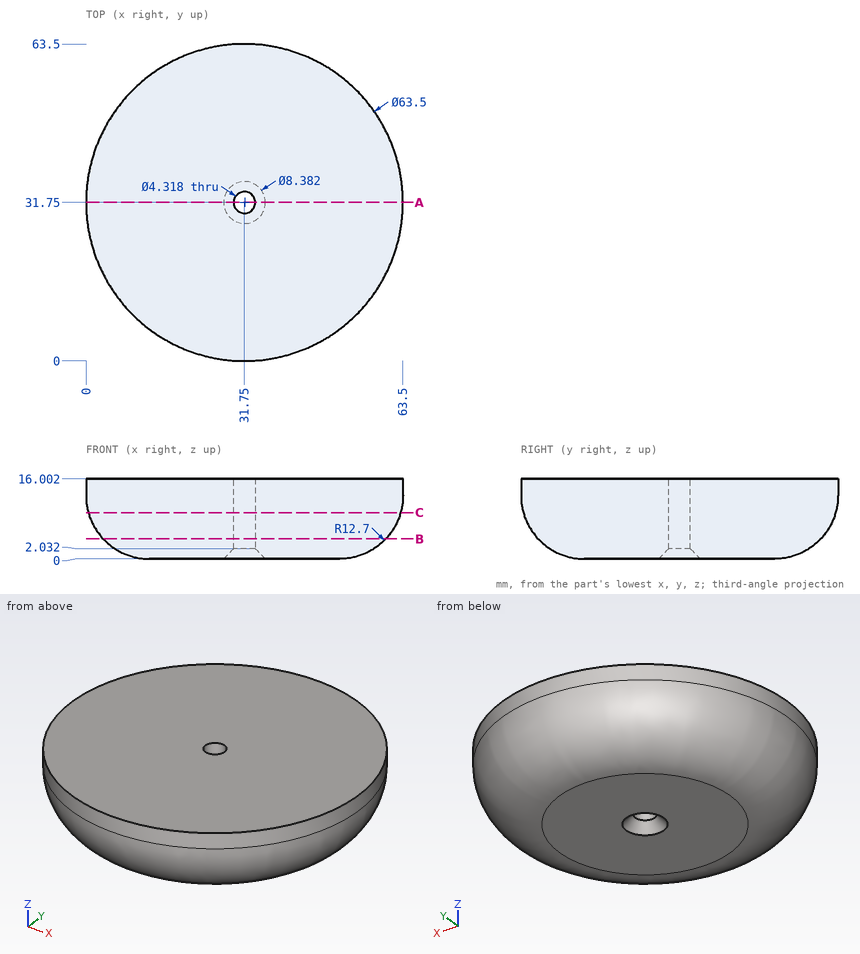
Answer from the drawing. Dimensions are ordinates in mm from the lowest x, y and z of the part. Give positions to 0.01 mm unless a question says otherwise; leave off trailing zeros. Loops run counter-clockwise (first coordinate to the right, second up) from the corner with the lowest first, then second, coordinate; pieces in that order, holes last. Notation, with made-up numbers: (-36.5, 44) -> (-4.5, 44) arc R15 cw to (-4.5, 62) -> close; hole circle Ø7 at (-35.75, 79). An arc over 180 degrees is marked (long way). Use a Markdown table: item, result.
Q1. Section B-B, the plane z = 4 is taken. Determine the outline of the cut face in (x, y), then the cut area to 3 significant figures.
Solved:
| item | result |
|---|---|
| outline | circle Ø56.6 at (31.75, 31.75); hole circle Ø4.32 at (31.75, 31.75) |
| area | 2,500 mm^2 |
Q2. Each of these flat-tipped pins is pushed along its axis until it touches: pin 1 (8 mm diameter, centred on x = 38.5, z = 2.5, fed in from +Y); pin 2 (8 mm diameter, centred on y = 21, z = 14, fed in from +X); pin 3 (3 mm diameter, centred on x = 9.5, y = 30, fed in from -Z). Where does it stop, or does it pass through?
Solved:
| item | result |
|---|---|
| pin 1 | stops at y = 61.26 |
| pin 2 | stops at x = 62.77 |
| pin 3 | stops at z = 0.12 |
Q3. Find the intervals of material crossed by line 1 along Y through (x, z) = (31.75, 12.5); line 2 along Y through (x, z) = (31.75, 6); line 3 along Z through (x, y) = (24, 5), in increasing order.
Solved:
| item | result |
|---|---|
| line 1 | y = 0 to 29.59, 33.91 to 63.5 |
| line 2 | y = 1.91 to 29.59, 33.91 to 61.59 |
| line 3 | z = 3.54 to 16 |
Q4. Section A-A, the plane y = 31.75 is taken. Determine the outline of the cut face in (x, z), then the cut area to 3 significant figures.
Solved:
| item | result |
|---|---|
| outline | (0, 12.7) arc R12.7 ccw to (12.7, 0) -> (27.56, 0) -> (29.59, 2.03) -> (29.59, 16) -> (0, 16) -> close; (33.91, 2.03) -> (35.94, 0) -> (50.8, 0) arc R12.7 ccw to (63.5, 12.7) -> (63.5, 16) -> (33.91, 16) -> close |
| area | 874 mm^2 |
Q5. Section C-C, the plane z = 9.25 is taken. Determine the outline of the cut face in (x, y).
Solved:
| item | result |
|---|---|
| outline | circle Ø62.54 at (31.75, 31.75); hole circle Ø4.32 at (31.75, 31.75) |
